Print and shaded views of the part. All mm, measured from the part's lowest x, y and z. A direction names the side the tool comes from. Round coordinates to 2 decimals unless told otherwise and drop trailing zeros. Write each loop counter-clockwise with the first axis right and the second up, starting at its lowest first coordinate (ties: lowest second). Pieces come first, ordered by that corner, then holes. Notation, with made-up numbers: M 48,73 L 82,73 A11 ccw 82,87 Z; hole C 31.25,39.5 d6. An arc over 180 degrees is marked long. Write item = value, one per line. Start each with the question number.
Q1. Drop flat-ended pins along their axis: P1, Ø10, axis at x = 39.5, z = 13, coming from the +Y side (1 decimal); P2, Ø3, axis at x = 85, z = 16.5, coming from the +Y side; P3, Ø7, axis at x = 43, z = 14, coming from the +Y side; P4, Ø10, axis at x = 55.5, y = 8.5, coming from the -Z side. Give the stop position or say it passes through.
Q2. Probe L1, parallel to X at y = 8, z = 22; L2, parallel to Y at x = 44.5, z = 4; L3, parallel to Y at x = 27.5, z = 22.5. List the from-to ranges inside material, lowest first.
Q3. Pull direction X, two halves, no side cores. Call the marked faces 1, 2, 3 and 4: released by +X, released by -X, zero draft, split by the parting line, or undercut.
Q4. Band-saw the part on D-D on y = 69. Write the cut outline in (x, z).
Q5. Tool access for the marked faces 5 and 6: list every direction of +Z, -Z, +X, -X, +Y, -Y with a clear straight run to the whole face (end or side of a thin tool).
Q6. Band-saw the part on B-B on y = 20. Write the cut outline in (x, z).
Q7. Band-saw the part on A-A on z = 11. Write the cut outline in (x, y) (1 decimal).
Q8. Band-saw the part on C-C on x = 44.5. Write the cut outline in (y, z), plus the area to 3 significant figures.
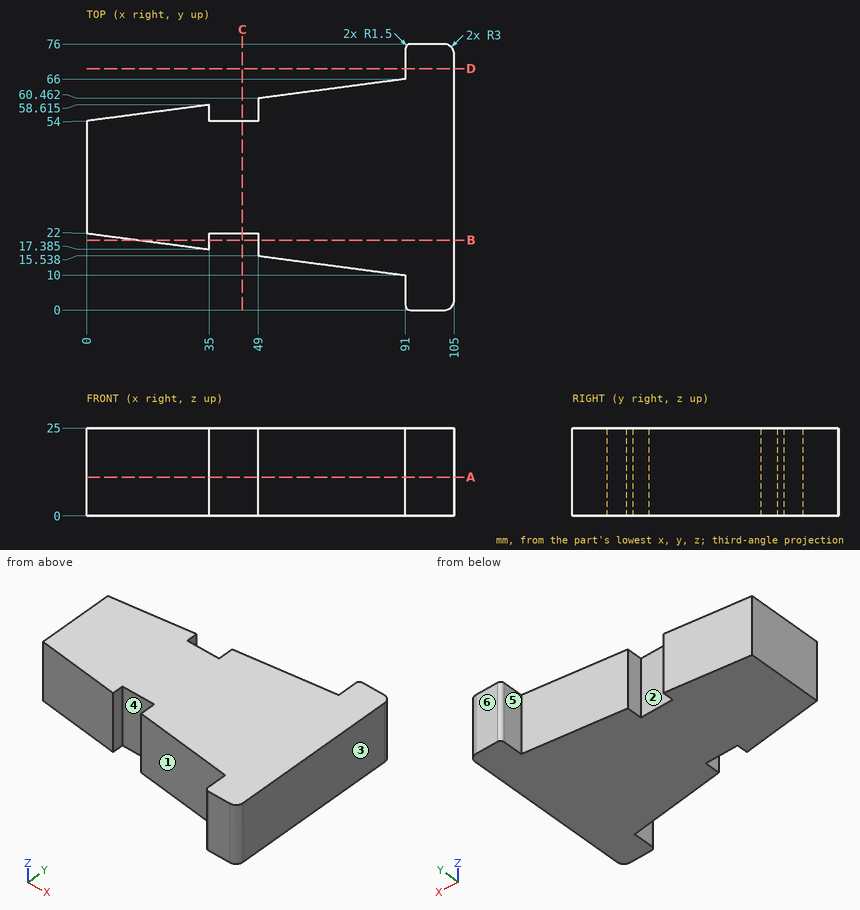
Conclusion:
q1.P1 = 58.6
q1.P2 = 65.41
q1.P3 = 54
q1.P4 = through
q2.L1 = 91 to 105
q2.L2 = 22 to 54
q2.L3 = 18.37 to 57.63
q3.face_1 = released by -X
q3.face_2 = undercut
q3.face_3 = released by +X
q3.face_4 = undercut
q4.outline = M 91,0 L 105,0 L 105,25 L 91,25 Z
q5.face_5 = +Z, -Z, -X, +Y
q5.face_6 = +Z, -Z, +X, -X, +Y
q6.outline = M 15.17,0 L 35,0 L 35,25 L 15.17,25 Z; M 49,0 L 105,0 L 105,25 L 49,25 Z
q7.outline = M 0,22 L 35,17.4 L 35,22 L 49,22 L 49,15.5 L 91,10 L 91,1.5 A1.5 ccw 92.5,0 L 102,0 A3 ccw 105,3 L 105,73 A3 ccw 102,76 L 92.5,76 A1.5 ccw 91,74.5 L 91,66 L 49,60.5 L 49,54 L 35,54 L 35,58.6 L 0,54 Z
q8.outline = M 22,0 L 54,0 L 54,25 L 22,25 Z
q8.area = 800 mm^2
